Read the model definition and answer for the solid it produces. Units are mm, in the model's axes. Face numbers are marked on the shaded views. A direction names the side the tool comes from. Coordinates: 2 decimals unless noted, no trailing zeros. Write each loop counter-clockwise with the first axis right and the second up, starting at its lowest first coordinate (ties: lowest second). Pieces come first, ordered by that corner, then holes.
1) Find the intervals of material crossed by line 1 (Z direction, x = -15, y = 9.5); line 2 (X direction, y = 10, z = -29.5); line 3 (Y direction, x = 38, z = 39.5), in increasing order.
2) Each of these flat-tipped pins is pushed along its axis until it touches: pin 1 Ø1 at (x, y) = (-15.5, 27) entering from +Z; pin 2 Ø12.5 at (y, z) = (13.5, -37) entering from +X; pin 3 Ø8 at (x, y) = (-14, 8) entering from +Z. Where does it stop, or does it pass through?
3) Which of the six approach directions +Z, -Z, +X, -X, +Y, -Y give full straight-line access (tool end or side, diameter ignored) to the marked faces 4, 5, 6, 7 and 8?
4) The part is cut by section C-C (z = -21). Determine the outline of the cut face in (x, y), then the cut area to 3 significant figures.
5) The part is cut by section D-D (y = 15). Give the number of separate pieces and of enclosed holes in the cut face, then the cut area to 3 significant figures.
6) The part is cut by section A-A (z = -50.5). Determine the outline of the cut face in (x, y), then the cut area to 3 significant figures.
7) Determine the mould class of the marked faces 1, 2 and 3 for opening direction X: +X half, -X half, draft (parallel to the pull), parting line (faces both ways), or undercut.
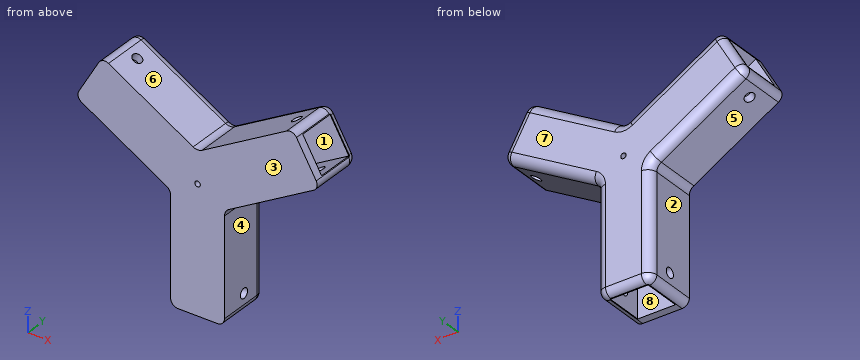
Autodesk Inventor part; units mm, degrees
ref_plane "YZ Plane" through (0, 0, 0) normal (1, 0, 0) x (0, 1, 0)
ref_plane "XZ Plane" through (0, 0, 0) normal (0, 1, 0) x (-1, 0, 0)
ref_plane "XY Plane" through (0, 0, 0) normal (0, 0, 1) x (1, 0, 0)
sketch "Sketch1" plane through (0, 0, 0) normal (0, 1, 0) x (-1, 0, 0)
  line L0 (0, 0) -> (30, 0)
  line L1 (30, 0) -> (30, -70)
  line L2 (30, -70) -> (0, -70)
  line L3 (0, -70) -> (0, 0)
  dimension "d0" = 30
  dimension "d1" = 70
extrude "Extrusion1" add sketch "Sketch1" along normal blind 30
sketch "Sketch6" plane through (0, 30, 0) normal (0, 1, 0) x (1, 0, 0)
  line L0 (0, 0) -> (-15, 0)
  line L1 (-30, 0) -> (0, 0)
  circle A0 centre (-15, 0) radius 1.5
  dimension "d32" = 3
extrude "Extrusion6" cut sketch "Sketch6" against normal blind 30
pattern_circular "Circular Pattern4" count 3 over 360 about axis through (-15, 30, 0) along (0, -1, 0) of "Extrusion1", "Extrusion6"
sketch "Sketch7" plane through (0, 0, -70) normal (0, 0, -1) x (-1, 0, 0)
  line L0 (4.5, 4.5) -> (25.5, 4.5)
  line L1 (25.5, 4.5) -> (25.5, 25.5)
  line L2 (25.5, 25.5) -> (4.5, 25.5)
  line L3 (4.5, 25.5) -> (4.5, 4.5)
  line L4 (15, 30) -> (15, 0)
  line L5 (4.5, 4.5) -> (25.5, 25.5) construction
  line L6 (25.5, 4.5) -> (4.5, 25.5) construction
  point P0 (0, 0)
  point P1 (15, 15)
  dimension "d38" = 21
  dimension "d39" = 21
extrude "Extrusion7" cut sketch "Sketch7" against normal blind 45
pattern_circular "Circular Pattern5" count 3 over 360 about axis through (-15, 30, 0) along (0, -1, 0) of "Extrusion7"
sketch "Sketch8" plane through (-15, 0, 17.3205) normal (-0.5, 0, 0.866) x (0.866, 0, 0.5)
  line L0 (61.3397, 0) -> (61.3397, 30)
  line L1 (61.3397, 15) -> (51.3397, 15)
  circle A0 centre (51.3397, 15) radius 2.75
  point P0 (4.3301, 0)
  dimension "d45" = 10
  dimension "d46" = 5.5
extrude "Extrusion8" cut sketch "Sketch8" against normal blind 30
pattern_circular "Circular Pattern6" count 3 over 360 about axis through (-15, 30, 0) along (0, -1, 0) of "Extrusion8"
fillet "Fillet5" radius 5 3 edges at (-15, 15, 17.3205) (0, 15, -8.6603) (-30, 15, -8.6603)
fillet "Fillet6" radius 5 6 edges at (-30, 30, -40.7735) (-57.8109, 30, 7.3964) (12.8109, 30, 33.3771) (-42.8109, 30, 33.3771) (27.8109, 30, 7.3964) (0, 30, -40.7735)
fillet "Fillet7" radius 4 15 edges at (-28.5355, 28.5355, -70) (-30, 12.5, -70) (-1.4645, 28.5355, -70) (0, 12.5, -70) (-15, 30, -70) (-68.854, 28.5355, 46.7221) (-68.1218, 12.5, 47.9904) (-82.3895, 28.5355, 23.2779) (-83.1218, 12.5, 22.0096) (-75.6218, 30, 35) (52.3895, 28.5355, 23.2779) (53.1218, 12.5, 22.0096) (38.854, 28.5355, 46.7221) (38.1218, 12.5, 47.9904) (45.6218, 30, 35)
properties part number "80_20_bot_connector"
Reported:
1. line 1: z = -25 to -1.5, 1.5 to 18.09
1. line 2: x = -30 to -25.5, -4.5 to 0
1. line 3: y = 0 to 4.5, 25.5 to 30
2. pin 1: stops at z = 17.9
2. pin 2: stops at x = 0
2. pin 3: stops at z = 20.21
3. face 4: -Z, +X, +Y, -Y
3. face 5: -Z, -X, +Y, -Y
3. face 6: +Z, +Y, -Y
3. face 7: +Z, -Z, +X, -X, +Y
3. face 8: -Z
4. outline: (-30, 0) - (0, 0) - (0, 25) arc R5 ccw to (-5, 30) - (-25, 30) arc R5 ccw to (-30, 25) - close
4. area: 889 mm2
5. separate pieces: 7
5. enclosed holes: 1
5. area: 2,900 mm2
6. outline: (-30, 0) - (0, 0) - (0, 25) arc R5 ccw to (-5, 30) - (-25, 30) arc R5 ccw to (-30, 25) - close; hole (-25.5, 4.5) - (-4.5, 4.5) - (-4.5, 25.5) - (-25.5, 25.5) - close
6. area: 448 mm2
7. face 1: undercut
7. face 2: -X half
7. face 3: draft
